The listing builds one solid part. Answer for the finished solid, in the listing's coordinates (mm). A direction names the side the tool comes from. Round coordinates to 2 decimals unless told otherwise and drop trailing zeros. Write each loop counter-clockwise with the first axis right and the second up, starting at its lowest first coordinate (ties: lowest second). Pieces come first, ordered by that corner, then holes. Notation, with made-up numbers: (75.5, -17.5) - (99.5, -17.5) arc R29 cw to (99.5, 19.5) - close; hole circle Ø7 at (77, 21). An arc over 180 degrees is marked (long way). Return JSON: item names as keys, results as strings. Group by question number.
(1) Section A-A, the plane x = 50 is taken. Write down the section's boundary in (y, z).
(2) Find the intervals of material crossed by line 1 along Y through (x, z) = (0, 6.5); line 2 along X through (y, z) = (25, 7.5); line 3 along Y through (x, z) = (47.5, 5.25), in increasing order. Write a range as [from, to].
(3) Which of the six approach directions +Z, -Z, +X, -X, +Y, -Y give full straight-line access (tool end or side, diameter ignored) to faces 4 (the flat face through (-1, -13, 10)), 5 (the flat face through (13, 0, 3))?
(4) Each of these flat-tipped pins is pushed along its axis until it touches: pin 1 (6 mm diameter, centred on x = 36.5, z = 6, fed in from -Y); pin 2 (0.9 mm diameter, centred on x = 12.5, z = 2, fed in from +Y); pin 3 (0.9 mm diameter, centred on x = -13.5, z = 2, fed in from +Y); pin 4 (5 mm diameter, centred on x = 0, y = 50, fed in from -Z). Where does it stop, or does it pass through?
(5) Determine the mould class of faces 1 (the flat face through (-1, -13, 0)), 2 (the cylindrical face through (-62.44, -2.75, 4.93)), 3 (the cylindrical face through (-1.33, 20.77, 4.93)) for opening direction X: +X half, -X half, draft (parallel to the pull), parting line (faces both ways), or undercut.
(6) Section D-D, the plane y = 0 is taken. Give the number of separate pieces and of enclosed holes in the cut face, then the cut area to 3 significant figures.
(7) Section B-B, the plane x = 0 is taken. Write down the section's boundary in (y, z), then the cut area to 3 significant figures.
Autodesk Fusion 360 part; units mm, degrees
sketch "Sketch3" plane through (0, 0, 0) normal (0, 0, 1) x (1, 0, 0)
  circle A0 centre (0, 0) radius 62.5
  dimension "d12" = 125
extrude "Extrude2" add sketch "Sketch3" along normal blind 10
sketch "Sketch4" plane through (0, 0, 10) normal (0, 0, 1) x (-1, 0, 0)
  circle A0 centre (0, 0) radius 62.5
  line L0 (0, 0) -> (0, -25)
  line L1 (0, -25) -> (0, -50)
  line L2 (0, 0) -> (25, 0)
  line L3 (25, 0) -> (50, 0)
  line L4 (0, 0) -> (-25, 0)
  line L5 (-25, 0) -> (-50, 0)
  line L6 (0, 0) -> (0, 25)
  line L7 (0, 25) -> (0, 50)
  point P0 (-25, 0)
  point P1 (25, 0)
  point P2 (0, -25)
  point P3 (0, -50)
  point P4 (-50, 0)
  point P5 (50, 0)
  point P6 (0, 50)
  point P7 (0, 25)
  dimension "d15" = 25
hole "Hole2" at (25, 0, 10) at (-25, 0, 10) at (0, 25, 10) direction (0, 0, -1) diameter 8.8646 end through all
hole "Hole3" at (0, 50, 10) at (50, 0, 10) at (0, -50, 10) at (-50, 0, 10) direction (0, 0, -1) diameter 6.4 end through all
hole "Hole4" at (0, 0, 10) direction (0, 0, -1) diameter 6.4 end through all countersink diameter 12.6 countersink angle 90
sketch "Sketch5" plane through (0, 0, 0) normal (0, 0, -1) x (1, 0, 0)
  circle A0 centre (0, 0) radius 3.2
  circle A1 centre (0, 50) radius 3.2
  circle A2 centre (0, -50) radius 3.2
  circle A3 centre (50, 0) radius 3.2
  circle A4 centre (-50, 0) radius 3.2
  circle A5 centre (25, 0) radius 4.4323
  circle A6 centre (-25, 0) radius 4.4323
  circle A7 centre (0, 0) radius 62.5
  line L0 (0, 0) -> (11.5, 0) construction
  line L1 (11.5, 0) -> (14.5, 0) construction
  line L2 (11.5, -3.125) -> (14.5, -3.125)
  line L3 (11.5, 3.125) -> (14.5, 3.125)
  line L4 (14.5, -3.125) -> (14.5, 3.125)
  line L5 (11.5, -3.125) -> (11.5, 3.125)
  circle A8 centre (0, -25) radius 4.4323
  line L6 (3.125, 11.5) -> (-3.125, 11.5)
  line L7 (3.125, 14.5) -> (-3.125, 14.5)
  line L8 (-3.125, 11.5) -> (-3.125, 14.5)
  line L9 (0, 11.5) -> (0, 14.5) construction
  line L10 (3.125, 11.5) -> (3.125, 14.5)
  line L11 (0, 0) -> (0, 11.5) construction
  line L12 (-11.5, 3.125) -> (-11.5, -3.125)
  line L13 (-14.5, 3.125) -> (-14.5, -3.125)
  line L14 (-11.5, -3.125) -> (-14.5, -3.125)
  line L15 (-11.5, 0) -> (-14.5, 0) construction
  line L16 (-11.5, 3.125) -> (-14.5, 3.125)
  line L17 (0, 0) -> (-11.5, 0) construction
  line L18 (-3.125, -11.5) -> (3.125, -11.5)
  line L19 (-3.125, -14.5) -> (3.125, -14.5)
  line L20 (3.125, -11.5) -> (3.125, -14.5)
  line L21 (0, -11.5) -> (0, -14.5) construction
  line L22 (-3.125, -11.5) -> (-3.125, -14.5)
  line L23 (0, 0) -> (0, -11.5) construction
  point P0 (0, 25)
  point P1 (-25, 0)
  point P2 (0, -25)
  dimension "d28" = 3
  dimension "d29" = 11.5
  dimension "d30" = 3.125
  dimension "d31" = -3.125
  dimension "d37" = 360
extrude "Extrude3" cut sketch "Sketch5" against normal blind 3 contours L2 L3 L4 L5 | L12 L13 L14 L16 | L18 L19 L20 L22
equation "thickness = 15 mm"
equation "height = 60 mm"
equation "hole_hole_dist = 25 mm"
equation "d30 = ( 6.25 / 2 ) * 1 mm"
equation "d31 = -d30"
Working result:
{
 "1": {"outline": "(-37.5, 0) - (-3.2, 0) - (-3.2, 10) - (-37.5, 10) - close; (3.2, 0) - (37.5, 0) - (37.5, 10) - (3.2, 10) - close"},
 "2": {"line 1": "y = [-62.5, -53.2], [-46.8, -3.2], [3.2, 20.57], [29.43, 46.8], [53.2, 62.5]", "line 2": "x = [-57.28, -4.43], [4.43, 57.28]", "line 3": "y = [-40.62, -2], [2, 40.62]"},
 "3": {"face 4": "+Z, +X, -X, +Y, -Y", "face 5": "-Z"},
 "4": {"pin 1": "stops at y = -52.76", "pin 2": "stops at y = 61.33", "pin 3": "stops at y = 61.12", "pin 4": "passes through"},
 "5": {"face 1": "draft", "face 2": "parting line", "face 3": "undercut"},
 "6": {"separate pieces": "6", "enclosed holes": "0", "area": "853 mm^2"},
 "7": {"outline": "(-62.5, 0) - (-53.2, 0) - (-53.2, 10) - (-62.5, 10) - close; (-46.8, 0) - (-3.2, 0) - (-3.2, 6.9) - (-6.3, 10) - (-46.8, 10) - close; (3.2, 0) - (11.5, 0) - (11.5, 3) - (14.5, 3) - (14.5, 0) - (20.57, 0) - (20.57, 10) - (6.3, 10) - (3.2, 6.9) - close; (29.43, 0) - (46.8, 0) - (46.8, 10) - (29.43, 10) - close; (53.2, 0) - (62.5, 0) - (62.5, 10) - (53.2, 10) - close", "area": "951 mm^2"}
}
